Part print with two shaded views. Sizes in mm from the minimum x, y, z corner. A direction names the side the tool comes from. Round coordinates to 2 decimals unless told otherwise and drop trailing zeros. Write each loop counter-clockwise with the first axis right and the second up, starting at its lowest first coordinate (ties: lowest second). Pieces come first, ordered by that corner, then holes. Notation, with made-up numbers: (73.25, 36) - (124.25, 36) arc R32 ccw to (124.25, 68) - close; hole circle Ø11 at (32, -5). An arc over 180 degrees is marked (long way). Use one line per item in the form item = value. Start each with the question number.
Item 1: Pull direction X, two halves, no side cores. Call the marked faces 1, 2 and 3: +X half, -X half, draft (parallel to the pull), parting line (faces both ways), or undercut.
Item 2: Pin check, flat tips, straight feed: pin 1 (6 mm diameter, centred on y = 12.5, z = 1.5, fed in from -X); pin 2 (5 mm diameter, centred on y = 11, z = 2, fed in from +X); pin 3 (10 mm diameter, centred on x = 21, y = 12, fed in from -Z). Stop position of each tip, or through.
Item 3: Band-saw the part on B-B, the plane y = 7. List the corners of the cut face in (x, z).
Item 4: Band-saw the part on C-C, the plane x = 5. List the corners of the cut face in (y, z).
Item 5: Tool access for the marked faces 4 and 5: list every direction of +Z, -Z, +X, -X, +Y, -Y with a clear straight run to the whole face (end or side of a thin tool).
Item 6: Band-saw the part on D-D, the plane x = 20.75. List the corners of the cut face in (y, z), and give its area (3 significant figures).
Item 7: Band-saw the part on A-A, the plane z = 5. List the corners of the cut face in (x, y).
Item 8: Drill centre lines: L1, parallel to Y at x = 21.75, z = 2; L2, parallel to X at y = 8.75, z = 5.5; L3, parallel to X at y = 10.5, z = 6. Where is each one in solid material? Low to high.
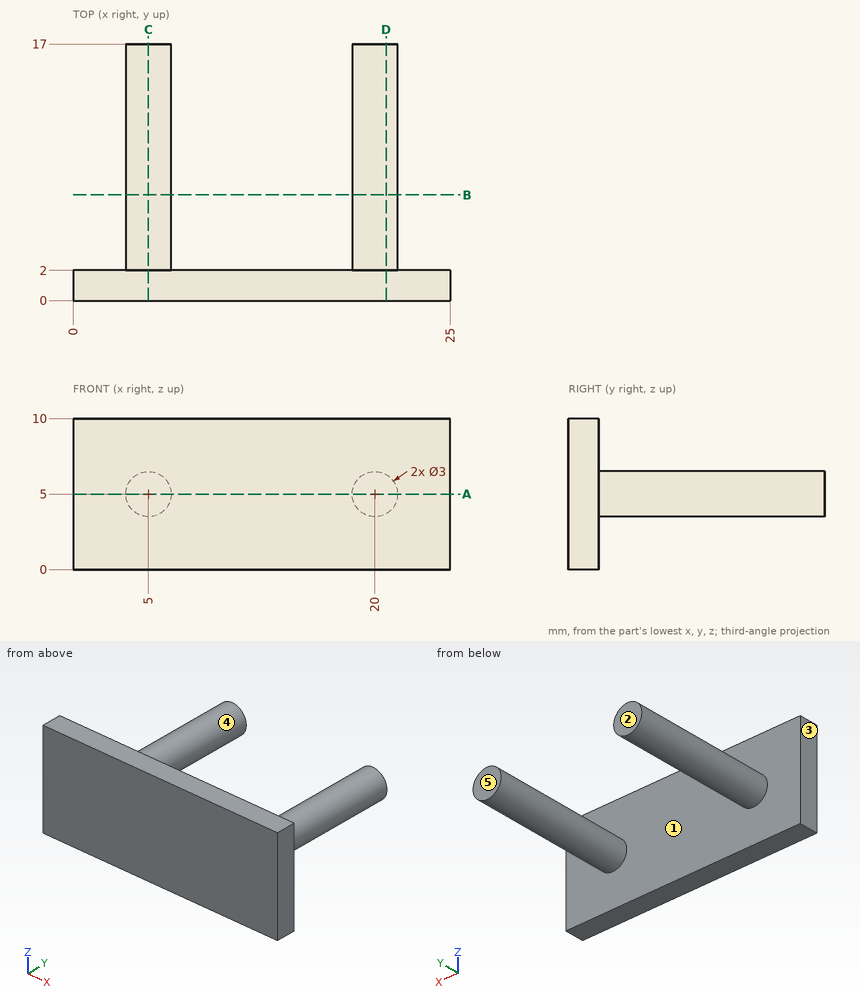
Determined:
q1.face_1 = undercut
q1.face_2 = draft
q1.face_3 = -X half
q2.pin_1 = 3.59
q2.pin_2 = 21.41
q2.pin_3 = 3.5
q3.outline = circle Ø3 at (5, 5); circle Ø3 at (20, 5)
q4.outline = (0, 0) - (2, 0) - (2, 3.5) - (17, 3.5) - (17, 6.5) - (2, 6.5) - (2, 10) - (0, 10) - close
q5.face_4 = +Y
q5.face_5 = +Z, -Z, +X, -X, +Y
q6.outline = (0, 0) - (2, 0) - (2, 3.7) - (17, 3.7) - (17, 6.3) - (2, 6.3) - (2, 10) - (0, 10) - close
q6.area = 59.0 mm²
q7.outline = (0, 0) - (25, 0) - (25, 2) - (21.5, 2) - (21.5, 17) - (18.5, 17) - (18.5, 2) - (6.5, 2) - (6.5, 17) - (3.5, 17) - (3.5, 2) - (0, 2) - close
q8.L1 = 0 to 2
q8.L2 = 3.59 to 6.41, 18.59 to 21.41
q8.L3 = 3.88 to 6.12, 18.88 to 21.12
